```python
from build123d import *

# Parameters (mm, degrees)
SKETCH1_R           = 6.65
SKETCH1_R_2         = 1.25
BOSS_EXTRUDE1_DEPTH = 4
SKETCH2_R           = 1.5
CUT_EXTRUDE1_DEPTH  = 5


with BuildPart() as part:
    # Sketch1 → Boss-Extrude1 (new body)
    with BuildSketch(Plane.XY):
        Polygon((22, 12.5), (22, -12.5), (12.5, -22), (-22, -22), (-22, 22), (12.5, 22), align=None)
        with Locations((8, 0)):
            Circle(SKETCH1_R, mode=Mode.SUBTRACT)
        with Locations((17, 9)):
            Circle(SKETCH1_R_2, mode=Mode.SUBTRACT)
        with Locations((17, -9)):
            Circle(SKETCH1_R_2, mode=Mode.SUBTRACT)
        with Locations((-16, 9)):
            Circle(SKETCH1_R_2, mode=Mode.SUBTRACT)
        with Locations((-16, -9)):
            Circle(SKETCH1_R_2, mode=Mode.SUBTRACT)
    extrude(amount=BOSS_EXTRUDE1_DEPTH)

    # Sketch2 → Cut-Extrude1 (cut, through all)
    with BuildSketch(Plane.XY.offset(4)):
        with Locations((-17, -19)):
            Circle(SKETCH2_R)
        with Locations((8.428932188, -19)):
            Circle(SKETCH2_R)
        with Locations((-17, 19)):
            Circle(SKETCH2_R)
        with Locations((8.428932188, 19)):
            Circle(SKETCH2_R)
    extrude(amount=-CUT_EXTRUDE1_DEPTH, mode=Mode.SUBTRACT)


solid = part.part
```
Part model, mm, in its own coordinate system. Give positions to 0.01 mm unless a question says otherwise; leave off trailing zeros. Order: outer loops, then holes, each group sorted by start corner. A loop starts at its lowest first (then second) coordinate and runs counter-clockwise, first axis right, second up. Notation, with made-up numbers: (-15, 62.25) - (-6, 62.25) arc R25 cw to (-6, 100.25) - close; hole circle Ø9 at (42, -10.75). An arc over 180 degrees is marked (long way). Use one line per item in the form item = value.
Item 1: Probe probe 1 along Y at (x, z) = (17, 3.05); probe 2 along X at (y, z) = (9.5, 2.95); probe 3 along Y at (x, z) = (-16, 1.95). List the from-to ranges inside material, lowest first. Write a range as from..to.
Solution:
probe_1 = -17.5..-10.25, -7.75..7.75, 10.25..17.5
probe_2 = -22..-17.15, -14.85..15.85, 18.15..22
probe_3 = -22..-20.12, -17.88..-10.25, -7.75..7.75, 10.25..17.88, 20.12..22
Item 2: Pin check, flat tip, straight feed: pin 1 Ø2.5 at (x, y) = (-17, -19) entering from +Z. Stop position of the tip, or through.
Solution:
pin_1 = through
Item 3: Slice it at D-D on z = 2.55. Count the separate pieces of the cut face and the enclosed holes in it, and give its area (3 significant figures).
Solution:
separate_pieces = 1
enclosed_holes = 9
area = 1,660 mm2
Item 4: Slice it at C-C on x = 14. Give the cut face in (y, z), and give its area (3 significant figures).
Solution:
outline = (-20.5, 0) - (-2.87, 0) - (-2.87, 4) - (-20.5, 4) - close; (2.87, 0) - (20.5, 0) - (20.5, 4) - (2.87, 4) - close
area = 141 mm2
Item 5: Two-plate mould, pull along X, no slides. Class faces 1 (the face through (-22, 0, 2)), 2 (the face through (0, 0, 4)), 3 (the face through (22, 0, 2)), 4 (the face through (16.84, 10.24, 1.97)): released by +X, released by -X, zero draft, split by the parting line, or undercut.
Solution:
face_1 = released by -X
face_2 = zero draft
face_3 = released by +X
face_4 = undercut
Item 6: Slice it at B-B on y = 0. Give the cut face in (x, z), and give its area (3 significant figures).
Solution:
outline = (-22, 0) - (1.35, 0) - (1.35, 4) - (-22, 4) - close; (14.65, 0) - (22, 0) - (22, 4) - (14.65, 4) - close
area = 123 mm2
Item 7: Slice it at A-A on y = 19. Give the cut face in (x, z).
Solution:
outline = (-22, 0) - (-18.5, 0) - (-18.5, 4) - (-22, 4) - close; (-15.5, 0) - (6.93, 0) - (6.93, 4) - (-15.5, 4) - close; (9.93, 0) - (15.5, 0) - (15.5, 4) - (9.93, 4) - close
